Part model, mm, in its own coordinate system. Round coordinates to 2 decimals unless told otherwise and drop trailing zeros. Loops run counter-clockwise (first coordinate to the right, second up) from the corner with the lowest first, then second, coordinate; pieces in that order, holes last.
1) Mould opens along Y. For faces 1 (the cylindrical face through (7.381, -27.36, 17.008)), 2 (the cylindrical face through (-22.498, -28.128, 25.35)), 3 (the cylindrical face through (-27.34, -36.6, 24.65)) say: +Y half, -Y half, draft (parallel to the pull), parting line (faces both ways), or undercut.
2) Probe line 1 (Z direction, x = -10, y = -21.5); line 2 (Y direction, x = -20, z = 35); line 3 (X direction, y = -23.75, z = 35). List the from-to ranges inside material, lowest first.
3) Band-saw the part on B-B, the plane z = 17. Write the cut outline in (x, y).
4) Band-saw the part on A-A, the plane x = 20. Write the cut outline in (y, z), then the cut area to 3 significant figures.
5) Band-saw the part on D-D, the plane y = -21. Write the cut outline in (x, z).
6) Band-saw the part on C-C, the plane x = -10. Write the cut outline in (y, z).
from build123d import *

# Parameters (mm, degrees)
BOSS_EXTRUDE1_DEPTH     = 50
TAP_DRILL_FOR_M6_TAP1_D = 5
M6_CLEARANCE_HOLE1_D    = 6.6


with BuildPart() as part:
    # Sketch1 → Boss-Extrude1 (new body)
    with BuildSketch(Plane.XY):
        with BuildLine():
            Line((28.2, -17.5), (-28.2, -17.5))
            Line((-28.2, -17.5), (-28.2, -34.5))
            ThreePointArc((-28.2, -34.5), (-27.321320344, -36.621320344), (-25.2, -37.5))
            Line((-25.2, -37.5), (25.2, -37.5))
            ThreePointArc((25.2, -37.5), (27.321320343, -36.621320344), (28.2, -34.5))
            Line((28.2, -34.5), (28.2, -17.5))
        make_face()
    extrude(amount=BOSS_EXTRUDE1_DEPTH)

    # Tap Drill for M6 Tap1 (through all)
    with Locations(Plane(origin=(0, 0, 0), x_dir=(-1, 0, 0), z_dir=(0, 0, -1))):
        with Locations((-20, -27.5), (20, -28.237657735)):
            Hole(TAP_DRILL_FOR_M6_TAP1_D / 2)

    # M6 Clearance Hole1 (through all)
    with Locations(Plane(origin=(0, -37.5, 0), x_dir=(-1, 0, 0), z_dir=(0, -1, 0))):
        with Locations((10, -15), (-10, -35), (10, -35), (-10, -15)):
            Hole(M6_CLEARANCE_HOLE1_D / 2)


solid = part.part
Reported:
1. face 1: draft
1. face 2: undercut
1. face 3: -Y half
2. line 1: z = 0 to 11.7, 18.3 to 31.7, 38.3 to 50
2. line 2: y = -37.5 to -30.74, -25.74 to -17.5
2. line 3: x = -28.2 to -13.3, -6.7 to 6.7, 13.3 to 28.2
3. outline: (-28.2, -34.5) arc R3 ccw to (-25.2, -37.5) - (-12.62, -37.5) - (-12.62, -17.5) - (-28.2, -17.5) - close; (-7.38, -37.5) - (7.38, -37.5) - (7.38, -17.5) - (-7.38, -17.5) - close; (12.62, -37.5) - (25.2, -37.5) arc R3 ccw to (28.2, -34.5) - (28.2, -17.5) - (12.62, -17.5) - close; hole circle Ø5 at (-20, -28.24); hole circle Ø5 at (20, -27.5)
4. outline: (-37.5, 0) - (-30, 0) - (-30, 50) - (-37.5, 50) - close; (-25, 0) - (-17.5, 0) - (-17.5, 50) - (-25, 50) - close
4. area: 750 mm2
5. outline: (-28.2, 0) - (28.2, 0) - (28.2, 50) - (-28.2, 50) - close; hole circle Ø6.6 at (-10, 15); hole circle Ø6.6 at (-10, 35); hole circle Ø6.6 at (10, 15); hole circle Ø6.6 at (10, 35)
6. outline: (-37.5, 0) - (-17.5, 0) - (-17.5, 11.7) - (-37.5, 11.7) - close; (-37.5, 18.3) - (-17.5, 18.3) - (-17.5, 31.7) - (-37.5, 31.7) - close; (-37.5, 38.3) - (-17.5, 38.3) - (-17.5, 50) - (-37.5, 50) - close
